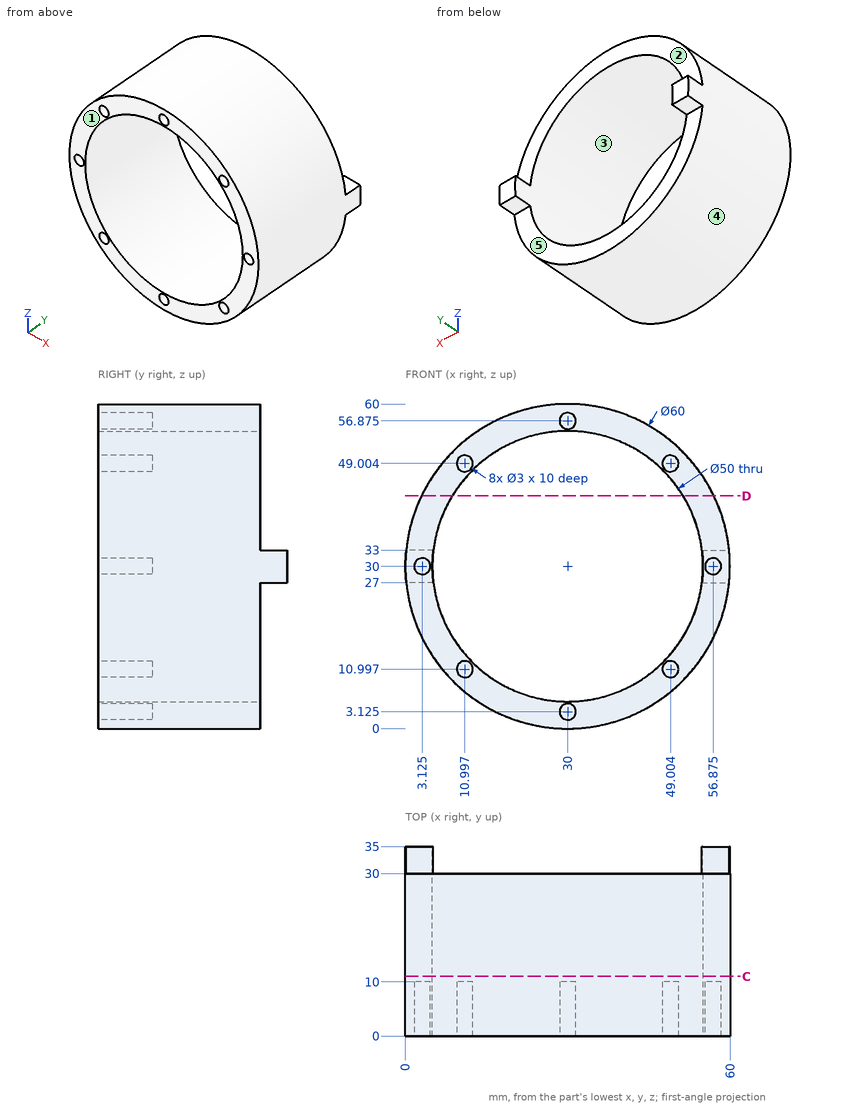
Could you check a few things on this drawing? It's one solid part, dimensions in mm from its lowest x, y, z. A direction names the side the tool comes from. Round coordinates to 2 decimals unless told otherwise and drop trailing zeros. Order: outer loops, then holes, each group sorted by start corner. A loop starts at its lowest first (then second) coordinate and runs counter-clockwise, first axis right, second up.
(1) I'm going to push flat-ended pins straight in: pin 1 (2.5 mm diameter, centred on x = 11, z = 11, fed in from -Y); pin 2 (8 mm diameter, centred on x = 32.5, y = 5.5, fed in from +Z); pin 3 (5 mm diameter, centred on x = 11, z = 11, fed in from +Y). Where does each tip first touch, or does it pass through?
Response values:
pin 1: stops at y = 10
pin 2: stops at z = 60
pin 3: stops at y = 30
(2) Imagine slicing it at C-C (y = 11). Write out the boundary of the cut face in (x, z).
Response values:
outline: circle Ø60 at (30, 30); hole circle Ø50 at (30, 30)
(3) If we mould it in two halves opening along X, with no side actions, what happens to the marked faces 3, 4 and 5? For each: released by +X, released by -X, zero draft, split by the parting line, or undercut.
Response values:
face 3: undercut
face 4: split by the parting line
face 5: zero draft
(4) Imagine slicing it at D-D (z = 43). Write out the boundary of the cut face in (x, y) (1 decimal), plus the area to 3 significant figures.
Response values:
outline: (3, 0) - (8.6, 0) - (8.6, 30) - (3, 30) - close; (51.4, 0) - (57, 0) - (57, 30) - (51.4, 30) - close
area: 341 mm2
(5) Please list where these lines run through material, in increasing order: line 1 along Z through (x, y) = (30, 6) (1 decimal); line 2 along Y through (x, z) = (5, 35); line 3 along Z through (x, y) = (30.5, 21.5) (1 decimal).
Response values:
line 1: z = 0 to 1.6, 4.6 to 5, 55 to 55.4, 58.4 to 60
line 2: y = 0 to 30
line 3: z = 0 to 5, 55 to 60
(6) Which directions (+Z, -Z, +X, -X, +Y, -Y) give clear straight access to the entire face, cutting with the end or side of a thin tool? Please do the marked faces 1 and 2.
Response values:
face 1: +Z, -Z, +X, -X, -Y
face 2: +Z, +X, -X, +Y
